Model file for the job. Use its own axes, mm. Round coordinates to 2 decimals unless told otherwise and drop trailing zeros. Loops run counter-clockwise (first coordinate to the right, second up) from the corner with the lowest first, then second, coordinate; pieces in that order, holes last. Notation, with made-up numbers: (62.25, 27) -> (104.25, 27) arc R35 cw to (104.25, 64) -> close; hole circle Ø2 at (18.25, -24.5). An arc over 180 degrees is marked (long way). Use a Markdown table: item, result.
from build123d import *

# Parameters (mm, degrees)
SKETCH_1_W          = 322.893717544
SKETCH_1_H          = 176.219773954
EXTRUDE_1_DEPTH     = 3
SKETCH_2_W          = 142.4
SKETCH_2_H          = 35
SKETCH_2_W_2        = 112.493717544
SKETCH_2_H_2        = 176.219773954
CUT_EXTRUDE_1_DEPTH = 3
SKETCH_4_W          = 142.4
SKETCH_4_H          = 18
CUT_EXTRUDE_2_DEPTH = 184.949559365
SKETCH_14_R         = 1.5
CUT_EXTRUDE_4_DEPTH = 184.949559365
EXTRUDE_3_DEPTH     = 3
CUT_EXTRUDE_5_DEPTH = 202.958956474
CUT_EXTRUDE_6_DEPTH = 202.958956474


with BuildPart() as part:
    # 草图1 → 凸台-拉伸1 (new body)
    with BuildSketch(Plane.XY):
        Rectangle(SKETCH_1_W, SKETCH_1_H)
    extrude(amount=EXTRUDE_1_DEPTH)

    # 草图2 → 切除-拉伸1 (cut)
    with BuildSketch(Plane.XY.offset(3)):
        with Locations((56.246858772, -70.609886977)):
            Rectangle(SKETCH_2_W, SKETCH_2_H)
        with Locations((-105.2, 0)):
            Rectangle(SKETCH_2_W_2, SKETCH_2_H_2)
    extrude(amount=-CUT_EXTRUDE_1_DEPTH, mode=Mode.SUBTRACT)

    # 草图4 → 切除-拉伸2 (cut, through all)
    with BuildSketch(Plane.XY.offset(3)):
        with Locations((56.246858772, -44.109886977)):
            Rectangle(SKETCH_4_W, SKETCH_4_H)
    extrude(amount=-CUT_EXTRUDE_2_DEPTH, mode=Mode.SUBTRACT)

    # 草图14 → 切除-拉伸4 (cut, through all)
    with BuildSketch(Plane.XY.offset(3)):
        with Locations((154.040490147, -60.609886977)):
            Circle(SKETCH_14_R)
        with Locations((154.040490147, -80.609886977)):
            Circle(SKETCH_14_R)
        with Locations((134.171700532, -60.609886977)):
            Circle(SKETCH_14_R)
        with Locations((134.171700532, -80.609886977)):
            Circle(SKETCH_14_R)
        with Locations((-21.677982988, -60.609886977)):
            Circle(SKETCH_14_R)
        with Locations((-21.677982988, -80.609886977)):
            Circle(SKETCH_14_R)
        with Locations((-41.546772603, -60.609886977)):
            Circle(SKETCH_14_R)
        with Locations((-41.546772603, -80.609886977)):
            Circle(SKETCH_14_R)
    extrude(amount=-CUT_EXTRUDE_4_DEPTH, mode=Mode.SUBTRACT)

    # 草图19 → 凸台-拉伸3 (add)
    with BuildSketch(Plane.XY.offset(3)):
        Polygon((-48.953141228, -34.8815165), (-48.953141228, 3.544050126), (-69.206772046, -34.8815165), align=None)
        Polygon((161.446858772, 3.544050126), (161.446858772, -34.8815165), (181.70048959, -34.8815165), align=None)
    extrude(amount=-EXTRUDE_3_DEPTH)

    # 草图20 → 切除-拉伸5 (cut, through all)
    with BuildSketch(Plane.XY.offset(3)):
        Polygon((-48.953141228, 3.544050126), (-48.953141228, 88.109886977), (161.446858772, 88.109886977), (161.446858772, 3.544050126), (138.622177289, 46.847462087), (-26.128459745, 46.847462087), align=None)
    extrude(amount=-CUT_EXTRUDE_5_DEPTH, mode=Mode.SUBTRACT)

    # 草图21 → 切除-拉伸6 (cut, through all)
    with BuildSketch(Plane.XY.offset(3)):
        Polygon((-69.206772046, -34.8815165), (-22.62920761, 46.919811864), (-26.128459745, 46.847462087), align=None)
        Polygon((181.70048959, -34.8815165), (135.122177289, 46.919811864), (138.622177289, 46.847462087), align=None)
    extrude(amount=-CUT_EXTRUDE_6_DEPTH, mode=Mode.SUBTRACT)


solid = part.part
Q1. Band-saw the part on B-B, the plane z = 1.5. Give the number of separate pieces and of enclosed holes in the cut face, plus the area to 3 significant figures.
Results list:
| item | result |
|---|---|
| separate pieces | 1 |
| enclosed holes | 8 |
| area | 20,300 mm² |
Q2. Band-saw the part on A-A, the plane y = -46.5. Give the cut face in (x, z), plus the area to 3 significant figures.
Results list:
| item | result |
|---|---|
| outline | (-48.95, 0) -> (-14.95, 0) -> (-14.95, 3) -> (-48.95, 3) -> close; (127.45, 0) -> (161.45, 0) -> (161.45, 3) -> (127.45, 3) -> close |
| area | 204 mm² |
Q3. Band-saw the part on D-D, the plane y = 21.5. Give the cut face in (x, z).
Results list:
| item | result |
|---|---|
| outline | (-37.1, 0) -> (149.6, 0) -> (149.6, 3) -> (-37.1, 3) -> close |
Q4. Drill centre lines: L1, parallel to Y at x = 42, z = 0.4; L2, parallel to X at y = -45.5, z = 1.25; L3, parallel to X at y = -81.5, z = 2.4. Where is each one in solid material? Low to high. Write a range as from..to.
Results list:
| item | result |
|---|---|
| L1 | y = -35.11..46.85 |
| L2 | x = -48.95..-14.95, 127.45..161.45 |
| L3 | x = -48.95..-42.75, -40.34..-22.89, -20.47..-14.95, 127.45..132.96, 135.38..152.83, 155.25..161.45 |
Q5. Band-saw the part on C-C, the plane x = 54. Give the cut face in (y, z).
Results list:
| item | result |
|---|---|
| outline | (-35.11, 0) -> (46.85, 0) -> (46.85, 3) -> (-35.11, 3) -> close |
Q6. Flat gauge pins, fed straight in: pin 1 (1.5 mm diameter, centred on y = -60.5, z = 1, fed in from -X); pin 2 (1.5 mm diameter, centred on x = -60, z = 2, fed in from -Y); pin 3 (1.5 mm diameter, centred on y = -71.5, z = 1, fed in from +X); pin 4 (2.5 mm diameter, centred on x = -41.55, y = -80.61, fed in from +Z). Where does each tip first touch, or does it go through?
Results list:
| item | result |
|---|---|
| pin 1 | stops at x = -48.95 |
| pin 2 | stops at y = -34.88 |
| pin 3 | stops at x = 161.45 |
| pin 4 | passes through |
